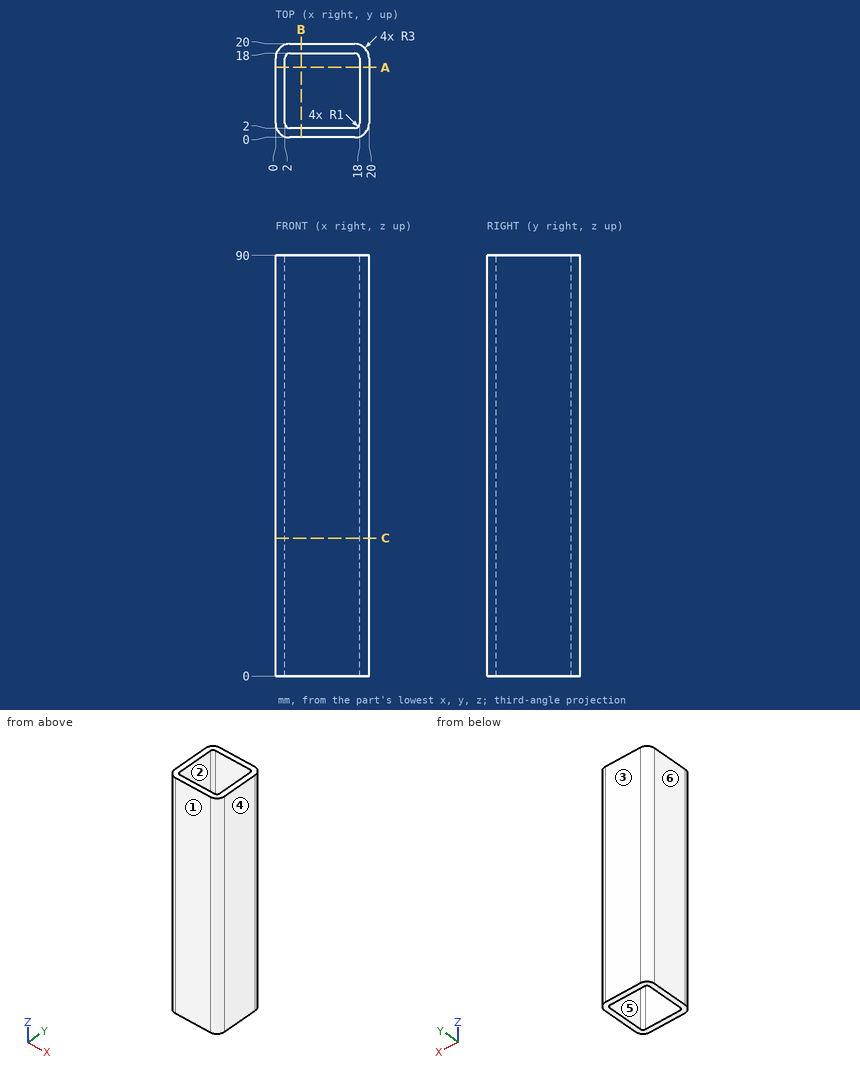
Here's the drawing with two shaded views (mm, measured from the low corner). I have some questions. A direction names the side the tool comes from. Coordinates: 2 decimals unless noted, no trailing zeros. Write each loop counter-clockwise with the first axis right and the second up, starting at its lowest first coordinate (ties: lowest second). Pieces come first, ordered by that corner, then holes. Notation, with made-up numbers: M -37,31.25 L -28,31.25 A8 ccw -28,44.25 Z; hole C 9,19 d9. An arc over 180 degrees is marked long. Answer as CSV lines item,"result".
Item 1: On a 3-axis mill with a long thin cutter (end or side, diameter ignored), from which of +Z, -Z, +X, -X, +Y, -Y can I reach the whole of each face in a straight line? I mean the marked faces 5 and 6. Say none if no direction works.
Geometry results:
face 5,"+Z, -Z"
face 6,"+Z, -Z, -X, +Y, -Y"
Item 2: We'd pull the mould along Y, two halves only. Please class the marked faces 1, 2, 3 and 4: +Y half, -Y half, draft (parallel to the pull), parting line (faces both ways), or undercut.
Geometry results:
face 1,"-Y half"
face 2,"undercut"
face 3,"+Y half"
face 4,"draft"
Item 3: Imagine slicing it at A-A on y = 15. List the corners of the cut face in (x, z) for me.
Geometry results:
outline,"M 0,0 L 2,0 L 2,90 L 0,90 Z; M 18,0 L 20,0 L 20,90 L 18,90 Z"
Item 4: Imagine slicing it at C-C on z = 29.5. List the corners of the cut face in (x, y) for me.
Geometry results:
outline,"M 0,3 A3 ccw 3,0 L 17,0 A3 ccw 20,3 L 20,17 A3 ccw 17,20 L 3,20 A3 ccw 0,17 Z; hole M 2,3 A1 ccw 3,2 L 17,2 A1 ccw 18,3 L 18,17 A1 ccw 17,18 L 3,18 A1 ccw 2,17 Z"
Item 5: I'm going to push a flat-ended pin straight in: P1, Ø6, axis at x = 6.5, y = 9.5, coming from the +Z side. Where does the tip first touch, or does it pass through?
Geometry results:
P1,"passes through"
Item 6: Please list where these lines run through material, in increasing order: line 1 along X through (y, z) = (16.75, 42); line 2 along X through (y, z) = (18.25, 65.5).
Geometry results:
line 1,"x = 0 to 2, 18 to 20"
line 2,"x = 0.27 to 19.73"
